```python
from build123d import *

# Parameters (mm, degrees)
SKETCH1_W           = 285
SKETCH1_H           = 71.5
BOSS_EXTRUDE1_DEPTH = 8
SKETCH2_W           = 35
SKETCH2_H           = 71.5
BOSS_EXTRUDE2_DEPTH = 12
CUT_EXTRUDE2_DEPTH  = 295.51188431
CHAMFER1_SIZE       = 10


with BuildPart() as part:
    # Sketch1 → Boss-Extrude1 (new body)
    with BuildSketch(Plane(origin=(0, 0, 0), x_dir=(1, 0, 0), z_dir=(0, 1, 0))):
        with Locations((142.5, 35.75)):
            Rectangle(SKETCH1_W, SKETCH1_H)
    extrude(amount=BOSS_EXTRUDE1_DEPTH)

    # Sketch2 → Boss-Extrude2 (add)
    with BuildSketch(Plane(origin=(0, 8, 0), x_dir=(1, 0, 0), z_dir=(0, 1, 0))):
        with Locations((17.5, 35.75)):
            Rectangle(SKETCH2_W, SKETCH2_H)
        with Locations((267.5, 35.75)):
            Rectangle(SKETCH2_W, SKETCH2_H)
    extrude(amount=BOSS_EXTRUDE2_DEPTH)

    # Sketch4 → Cut-Extrude2 (cut, through all)
    with BuildSketch(Plane.XZ):
        Polygon((0, -17), (44, -17), (52, -11), (233, -11), (241, -17), (285, -17), (285, 0), (0, 0), align=None)
        Polygon((44, -54.5), (52, -60.5), (233, -60.5), (241, -54.5), (285, -54.5), (285, -71.5), (0, -71.5), (0, -54.5), align=None)
    extrude(amount=-CUT_EXTRUDE2_DEPTH, mode=Mode.SUBTRACT)

    # Chamfer1
    chamfer1_edges = [part.edges().sort_by_distance(p)[0] for p in [
        (0, 0, -35.75),
        (285, 0, -35.75),
    ]]
    chamfer(chamfer1_edges, length=CHAMFER1_SIZE)


solid = part.part
```
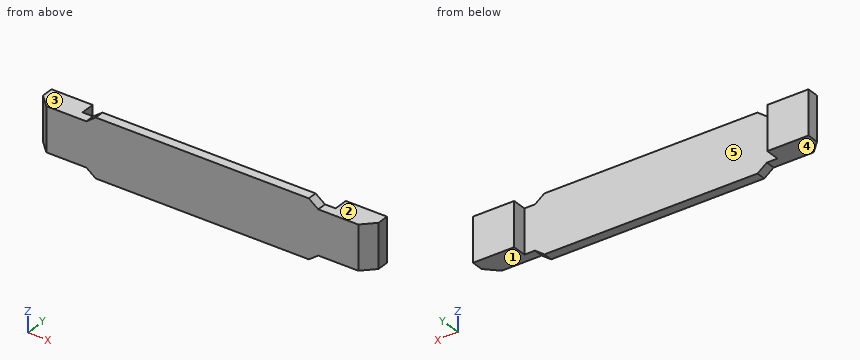
Input: part model. Units: mm. Frame: model coordinates. Face numbers are marked on the shaded views. A direction names the side the tool comes from. Coordinates: 2 decimals unless noted, no trailing zeros. Loops run counter-clockwise (first coordinate to the right, second up) from the corner with the lowest first, then second, coordinate; pieces in that order, holes last. Notation, with made-up numbers: M 89,5.25 L 112,5.25 A22 ccw 112,31.25 Z; hole C 63.25,2.5 d7. An arc over 180 degrees is marked long. Answer in a Markdown table with one row per item.
1. Material intervals for line 1 (X direction, y = 10.25, z = -28); line 2 (Y direction, x = 83, z = -56); line 3 (X direction, y = 8.25, z = -41), sorted ascending.
Response:
| item | result |
|---|---|
| line 1 | x = 0 to 35, 250 to 285 |
| line 2 | y = 0 to 8 |
| line 3 | x = 1.75 to 35, 250 to 283.25 |
2. Reachability of the marked faces 1, 2, 3, 4 and 5 from +Z, -Z, +X, -X, +Y, -Y: full face, straight path, thin tool, end or side. Return the list, or none.
Response:
| item | result |
|---|---|
| face 1 | -Z, +X, +Y, -Y |
| face 2 | +Z, +X, +Y, -Y |
| face 3 | +Z, -X, +Y, -Y |
| face 4 | -Z, -X, +Y, -Y |
| face 5 | +Z, -Z, +Y |
3. Section D-D, the plane x = 236. Output: boundary loops of the cut face in (y, z), then the cut area to 3 significant figures.
Response:
| item | result |
|---|---|
| outline | M 0,-58.25 L 8,-58.25 L 8,-13.25 L 0,-13.25 Z |
| area | 360 mm2 |
4. Section B-B, the plane z = -39. Output: boundary loops of the cut face in (x, y), then the cut area to 3 significant figures.
Response:
| item | result |
|---|---|
| outline | M 0,10 L 10,0 L 275,0 L 285,10 L 285,20 L 250,20 L 250,8 L 35,8 L 35,20 L 0,20 Z |
| area | 3,020 mm2 |
5. First-contact query: pin 1 (10 mm diameter, centred on x = 157, z = -53.5, fed in from +Y); pin 2 (10 mm diameter, centred on x = 239, y = 6, fed in from +Z); pin 3 (10 mm diameter, centred on x = 265.5, y = 13, fed in from -Z). Flat tips, straight axial feed; report the tip coordinate or a pass-through.
Response:
| item | result |
|---|---|
| pin 1 | stops at y = 8 |
| pin 2 | stops at z = -11.75 |
| pin 3 | stops at z = -54.5 |
6. Section A-A, the plane y = 12.5. Output: boundary loops of the cut face in (x, z), then the cut area to 4 significant figures.
Response:
| item | result |
|---|---|
| outline | M 0,-54.5 L 35,-54.5 L 35,-17 L 0,-17 Z; M 250,-54.5 L 285,-54.5 L 285,-17 L 250,-17 Z |
| area | 2,625 mm2 |
7. Section C-C, the plane x = 148.5. Output: boundary loops of the cut face in (y, z), then the cut area to 3 significant figures.
Response:
| item | result |
|---|---|
| outline | M 0,-60.5 L 8,-60.5 L 8,-11 L 0,-11 Z |
| area | 396 mm2 |
